Check sheet for the modelled part. Datum: model origin and axes. Units: mm. Face numbers are marked on the shaded views. A direction names the side the tool comes from. Round coordinates to 2 decimals unless told otherwise and drop trailing zeros. Loops run counter-clockwise (first coordinate to the right, second up) from the corner with the lowest first, then second, coordinate; pieces in that order, holes last. Notation, with made-up numbers: M -33.75,65.25 L -24.75,65.25 A13 ccw -24.75,77.25 Z; hole C 15.5,84 d7. An arc over 180 degrees is marked long. Write item = value, one per line. Start each with the question number.
(1) Cross-section at A-A on y = 8. Record the boundary of the cut face in (x, z).
(2) Go/stop test with a flat-tipped pin: P1, Ø3, axis at x = -10, y = -26.7, coming from the +Z side. Record where the tip stops, or that it passes through.
(3) Cross-section at D-D on y = 37.3. Record the boundary of the cut face in (x, z), plus the area to 3 significant figures.
(4) Cross-section at B-B on z = 14. Record the boundary of the cut face in (x, y), plus the area to 3 significant figures.
(5) Scan lines: L1, parallel to X at y = -1, z = 8; L2, parallel to Y at x = -10, z = 0.85; L3, parallel to Y at x = -1, z = 3.25. Record each from-to range of solid material in increasing order. Write a range as from..to.
(6) Cross-section at C-C on x = 10. Record the boundary of the cut face in (y, z), plus the area to 3 significant figures.
(7) Set-up check for the marked faces 1 and 2: record each of +Z, -Z, +X, -X, +Y, -Y from which the full face is reachable in a straight line by a thin tool's end or side.
(8) Mould release check, pull along X, two halves, no side actions. Record for the marked faces 3, 4 and 5: pulls with the +X half, pulls with the -X half, needs draft (parallel to the pull), parting line crosses it, or undercut.
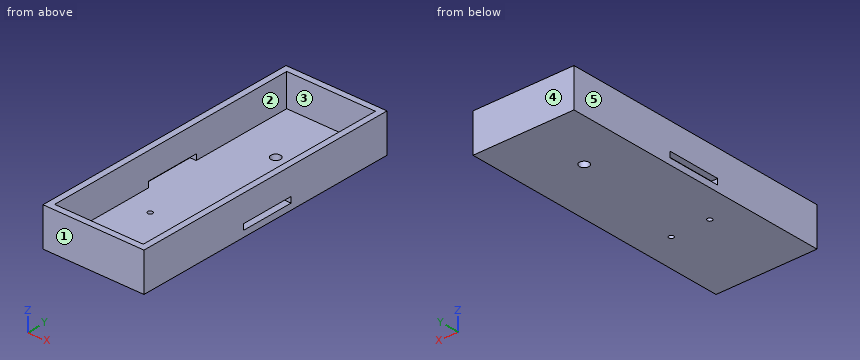
from build123d import *

# Parameters (mm, degrees)
F0_W          = 52.4
F0_H          = 142.4
F0_W_2        = 46
F0_H_2        = 136
F0_R          = 1.25
F0_R_2        = 2.5
F1_DEPTH      = 3.2
F2_DEPTH      = 20
F3_W          = 28
F3_H          = 3
F4_DEPTH      = 3.201
F4_DEPTH_BACK = 49.201


with BuildPart() as f1:
    # F0 (on Top) → F1 (new body)
    with BuildSketch(Plane.XY):
        Rectangle(F0_W, F0_H)
        Rectangle(F0_W_2, F0_H_2, mode=Mode.SUBTRACT)
        Rectangle(F0_W_2, F0_H_2)
        with Locations((-10, -26.7)):
            Circle(F0_R, mode=Mode.SUBTRACT)
        with Locations((10, -26.7)):
            Circle(F0_R, mode=Mode.SUBTRACT)
        with Locations((-1.5, 37.3)):
            Circle(F0_R_2, mode=Mode.SUBTRACT)
    extrude(amount=F1_DEPTH)

    # F0 (on Top) → F2 (join)
    with BuildSketch(Plane.XY):
        Rectangle(F0_W, F0_H)
        Rectangle(F0_W_2, F0_H_2, mode=Mode.SUBTRACT)
    extrude(amount=F2_DEPTH)

    # F3 (on face) → F4 (cut, two sides)
    with BuildSketch(Plane.YZ.offset(-23)) as f4_sk:
        with Locations((1, 4.7)):
            Rectangle(F3_W, F3_H)
    extrude(amount=-F4_DEPTH, mode=Mode.SUBTRACT)
    extrude(f4_sk.sketch, amount=F4_DEPTH_BACK, mode=Mode.SUBTRACT)


solid = f1.part
Result:
q1.outline = M -26.2,0 L 26.2,0 L 26.2,3.2 L -26.2,3.2 Z; M -26.2,6.2 L -23,6.2 L -23,20 L -26.2,20 Z; M 23,6.2 L 26.2,6.2 L 26.2,20 L 23,20 Z
q2.P1 = 3.2
q3.outline = M -26.2,0 L -4,0 L -4,3.2 L -23,3.2 L -23,20 L -26.2,20 Z; M 1,0 L 26.2,0 L 26.2,20 L 23,20 L 23,3.2 L 1,3.2 Z
q3.area = 259 mm^2
q4.outline = M -26.2,-71.2 L 26.2,-71.2 L 26.2,71.2 L -26.2,71.2 Z; hole M -23,-68 L 23,-68 L 23,68 L -23,68 Z
q4.area = 1,210 mm^2
q5.L1 = -26.2..-23, 23..26.2
q5.L2 = -71.2..-27.95, -25.45..71.2
q5.L3 = -71.2..-68, 68..71.2
q6.outline = M -71.2,0 L -27.95,0 L -27.95,3.2 L -68,3.2 L -68,20 L -71.2,20 Z; M -25.45,0 L 71.2,0 L 71.2,20 L 68,20 L 68,3.2 L -25.45,3.2 Z
q6.area = 555 mm^2
q7.face_1 = +Z, -Z, +X, -X, -Y
q7.face_2 = +Z
q8.face_3 = undercut
q8.face_4 = needs draft
q8.face_5 = pulls with the -X half
